Autodesk Inventor part; units mm, degrees
ref_plane "YZ Plane" through (0, 0, 0) normal (1, 0, 0) x (0, 1, 0)
ref_plane "XZ Plane" through (0, 0, 0) normal (0, 1, 0) x (-1, 0, 0)
ref_plane "XY Plane" through (0, 0, 0) normal (0, 0, 1) x (1, 0, 0)
sketch "スケッチ1" plane through (0, 0, 0) normal (0, 0, 1) x (1, 0, 0)
  circle A0 centre (0, 0) radius 11
  dimension "d0" = 22
extrude "押し出し1" add sketch "スケッチ1" along normal blind 5.5
sketch "スケッチ2" plane through (0, 0, 0) normal (0, 0, -1) x (-1, 0, 0)
  circle A0 centre (0, 0) radius 12
  dimension "d3" = 24
extrude "押し出し2" add sketch "スケッチ2" along normal blind 1.5
sketch "スケッチ3" plane through (0, 0, 5.5) normal (0, 0, 1) x (1, 0, 0)
  point P0 (0, 0)
  point P1 (0, 0)
hole "穴1" at (0, 0, 5.5) direction (0, 0, -1) diameter 8 depth 7 tip angle 118
properties part number "玉軸受2 F608ZZ"
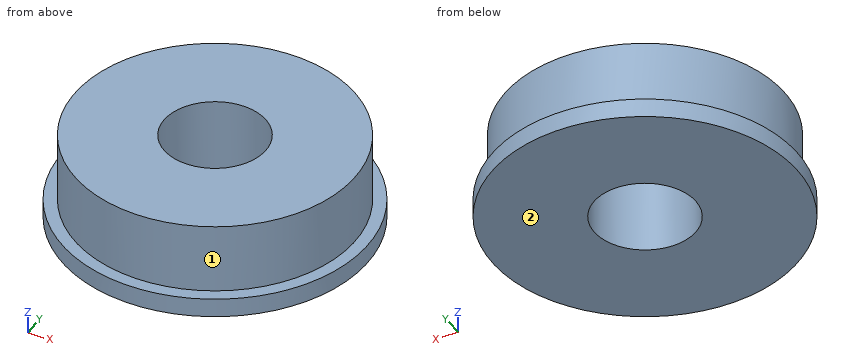
CAD build for the part. Positions are in the model's coordinates, mm. Face numbers are marked on the shaded views. A direction names the side the tool comes from. Round coordinates to 2 decimals unless told otherwise and drop trailing zeros. Loops run counter-clockwise (first coordinate to the right, second up) from the corner with the lowest first, then second, coordinate; pieces in that order, holes last. Notation, with made-up numbers: M -13,36.25 L 9,36.25 A31 cw 9,75.25 Z; hole C 34.25,67 d5. An arc over 180 degrees is marked long. Return JSON: item names as keys, results as strings. Group by question number.
(1) Saw through at A-A, the plane x = 0. List the corners of the cut face in (y, z).
(2) Tool access for the marked faces 1 and 2: list every direction of +Z, -Z, +X, -X, +Y, -Y with a clear straight run to the whole face (end or side of a thin tool).
(3) Saw through at D-D, the plane x = -6. List the corners of the cut face in (y, z).
(4) Saw through at C-C, the plane z = 1.5. List the corners of the cut face in (x, y), and give its area (3 significant figures).
(5) Wall check: probe 1 along Y at (x, z) = (0, 2.25); probe 2 along X at (y, z) = (0.5, 3.5); probe 3 along Y at (x, z) = (-3, 4.5). Give the ranges that are in metal, low to high. Write a range as [from, to].
(6) Drop flat-ended pins along their axis: P1, Ø2, axis at x = 7, z = 5, coming from the -Y side; P2, Ø4, axis at y = -3, z = -0.5, coming from the -X side. Give the stop position or say it passes through.
Answer list:
{
 "1": {"outline": "M -12,-1.5 L -4,-1.5 L -4,5.5 L -11,5.5 L -11,0 L -12,0 Z; M 4,-1.5 L 12,-1.5 L 12,0 L 11,0 L 11,5.5 L 4,5.5 Z"},
 "2": {"face 1": "+Z", "face 2": "-Z, +X, -X, +Y, -Y"},
 "3": {"outline": "M -10.39,-1.5 L 10.39,-1.5 L 10.39,0 L 9.22,0 L 9.22,5.5 L -9.22,5.5 L -9.22,0 L -10.39,0 Z"},
 "4": {"outline": "C 0,0 d22; hole C 0,0 d8", "area": "330 mm2"},
 "5": {"probe 1": "[-11, -4], [4, 11]", "probe 2": "[-10.99, -3.97], [3.97, 10.99]", "probe 3": "[-10.58, -2.65], [2.65, 10.58]"},
 "6": {"P1": "y = -9.22", "P2": "x = -11.96"}
}
